```python
from build123d import *

# Parameters (mm, degrees)
F0_W      = 50.8
F0_H      = 50.8
F1_FACE_W = 50.8
F1_FACE_H = 50.8


# Not quite as in the source:
# - an extrude whose draft closes it to a point is written as a loft to that point


with BuildPart() as f1:
    # F0 (on Front) → F1 section 0
    with BuildSketch(Plane.XZ, mode=Mode.PRIVATE) as f1_s0:
        Rectangle(F0_W, F0_H)
    loft([f1_s0.sketch, Vertex(0, -62.8672060768, 0)], ruled=True)

    # F1_face (on face) → F2 section 0
    with BuildSketch(Plane(origin=(0, 0, 0), x_dir=(1, 0, 0), z_dir=(0, 1, 0)), mode=Mode.PRIVATE) as f2_s0:
        Rectangle(F1_FACE_W, F1_FACE_H)
    loft([f2_s0.sketch, Vertex(0, 14.6646968374, 0)], ruled=True)


solid = f1.part
```
Source: CAD feature listing. Evaluate the final solid. Frame: model axes, mm. Round coordinates to 2 decimals unless told otherwise and drop trailing zeros. Order: outer loops, then holes, each group sorted by start corner. A loop starts at its lowest first (then second) coordinate and runs counter-clockwise, first axis right, second up. Notation, with made-up numbers: (-2.75, -33) -> (25.25, -33) arc R14 cw to (25.25, -18) -> close; hole circle Ø1 at (51, 63). An arc over 180 degrees is marked (long way). Use CSV: the item, a comma, the result in double quotes.
(1) First-contact query: pin 1 Ø5 at (x, y) = (10, -22.5) entering from +Z; pin 2 Ø2 at (y, z) = (-13, -12.5) entering from -X; pin 3 Ø1 at (x, y) = (-8.5, -6) entering from -Z. Flat tips, straight axial feed; report the tip coordinate or a pass-through.
Report:
pin 1,"z = 17.32"
pin 2,"x = -20.55"
pin 3,"z = -23.18"
(2) Section D-D on y = -47.5. Return the cut outline in (x, z).
Report:
outline,"(-6.21, -6.21) -> (6.21, -6.21) -> (6.21, 6.21) -> (-6.21, 6.21) -> close"
(3) Section C-C on y = -16.5. Return the cut outline in (x, z), and give its area (3 significant figures).
Report:
outline,"(-18.73, -18.73) -> (18.73, -18.73) -> (18.73, 18.73) -> (-18.73, 18.73) -> close"
area,"1,400 mm^2"
(4) Section A-A on z = -8.5. Return the cut outline in (x, y), and give its area (3 significant figures).
Report:
outline,"(-25.4, 0) -> (-8.5, -41.83) -> (8.5, -41.83) -> (25.4, 0) -> (8.5, 9.76) -> (-8.5, 9.76) -> close"
area,"1,750 mm^2"
(5) Ray query, L1, parallel to Y at x = -22.5, z = 6.5; L2, parallel to Y at x = 14, z = 16; L3, parallel to Z at x = -9.5, y = -4.5. Return the intervals inside material, ascending.
Report:
L1,"-7.18 to 1.67"
L2,"-23.27 to 5.43"
L3,"-23.58 to 23.58"
(6) Section B-B on x = 7.5. Return the cut outline in (y, z).
Report:
outline,"(-44.3, -7.5) -> (0, -25.4) -> (10.33, -7.5) -> (10.33, 7.5) -> (0, 25.4) -> (-44.3, 7.5) -> close"
